Check sheet for the modelled part. Datum: model origin and axes. Units: mm. Face numbers are marked on the shaded views. A direction names the side the tool comes from. Coordinates: 2 decimals unless noted, no trailing zeros. Write each loop counter-clockwise with the first axis right and the second up, starting at its lowest first coordinate (ties: lowest second). Pieces come first, ordered by that corner, then holes. Notation, with made-up numbers: (35.25, 47) - (60.25, 47) arc R26 cw to (60.25, 75) - close; hole circle Ø3 at (18.5, -17). An arc over 180 degrees is marked (long way). Answer as CSV lines item,"result". Start each with the question number.
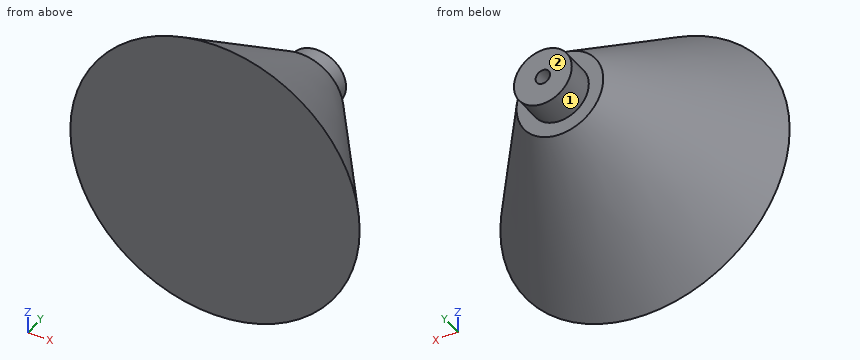
Autodesk Fusion 360 part; units mm, degrees
sketch "Sketch1" plane through (0, 0, 0) normal (0, 1, 0) x (1, 0, 0)
  circle A0 centre (0, 0) radius 50
  dimension "d1" = 100
extrude "Extrude1" add sketch "Sketch1" along normal blind 50 draft -35 makes body 1
sketch "Sketch2" plane through (0, 50, 0) normal (0, 1, 0) x (-1, 0, 0)
  circle A0 centre (0, 0) radius 14.9896
sketch "Sketch3" plane through (0, 50, 0) normal (0, 1, 0) x (-1, 0, 0)
  circle A0 centre (0, 0) radius 10
  dimension "d5" = 20
extrude "Extrude2" add sketch "Sketch3" along normal blind 10 bodies 1
sketch "Sketch4" plane through (0, 60, 0) normal (0, 1, 0) x (-1, 0, 0)
  circle A0 centre (0, 0) radius 10
  circle A1 centre (0, 0) radius 2.4995
  dimension "d8" = 4.999
extrude "Extrude3" cut sketch "Sketch4" against normal blind 5 contours A1 bodies 1
copy_body "Body->Comp1" bodies 1 removing the originals makes body 2 in component "Component"
component "Component" placed x (1, 0, 0) y (0, 1, 0) z (0, 0, 1) at (0, 0, 0)
(1) Go/stop test with flat-tipped pins: P1, Ø8, axis at x = -15.5, y = 11.5, coming from the -Z side; P2, Ø1, axis at x = -25.5, y = 27, coming from the -Z side; P3, Ø4, axis at x = 29, z = 20, coming from the +Y side. Record where each tip stops, or that it passes through.
(2) Cross-section at B-B on z = 0. Record the boundary of the cut face in (x, y), plus the area to 3 significant figures.
(3) Cross-section at A-A on x = 0. Record the boundary of the cut face in (y, z).
(4) Material ranges on probe 1 along Z at (x, y) = (0, 57); probe 2 along Y at (x, z) = (1, 10); probe 3 along X at (y, z) = (31.5, 6), recorded low to high. Write a range as from..to.
(5) Tool access check on the marked faces 1 and 2. Record the directions out of +Z, -Z, +X, -X, +Y, -Y that give a thin tool (end or side, any length) a straight path to the whole face; none if there is none.
Checked values:
1,P1,"z = -42.29"
1,P2,"z = -18.71"
1,P3,"y = 23.95"
2,outline,"(-50, 0) - (50, 0) - (14.99, 50) - (10, 50) - (10, 60) - (2.5, 60) - (2.5, 55) - (-2.5, 55) - (-2.5, 60) - (-10, 60) - (-10, 50) - (-14.99, 50) - close"
2,area,"3,420 mm^2"
3,outline,"(0, -50) - (50, -14.99) - (50, -10) - (60, -10) - (60, -2.5) - (55, -2.5) - (55, 2.5) - (60, 2.5) - (60, 10) - (50, 10) - (50, 14.99) - (0, 50) - close"
4,probe 1,"-10..-2.5, 2.5..10"
4,probe 2,"0..50"
4,probe 3,"-27.29..27.29"
5,face 1,"+Y"
5,face 2,"+Z, -Z, +X, -X, +Y"
